Model file for the job. Use its own axes, mm. A direction names the side the tool comes from. Coordinates: 2 decimals unless noted, no trailing zeros. Write each loop counter-clockwise with the first axis right and the second up, starting at its lowest first coordinate (ties: lowest second). Pieces come first, ordered by that corner, then holes. Notation, with made-up numbers: (-16.75, 16.5) -> (-4.75, 16.5) arc R11 cw to (-4.75, 20.5) -> close; hole circle Ø4 at (59, 44). An arc over 180 degrees is marked (long way). Answer as a JSON object with one key per item and string values. Group by question number.
from build123d import *

# Parameters (mm, degrees)
SKETCH2_W                = 12.7
SKETCH2_H                = 12.7
BOSS_EXTRUDE4_DEPTH      = 3.6068
BOSS_EXTRUDE4_DEPTH_BACK = 2.7686
SKETCH3_W                = 1.000000006
SKETCH3_H                = 3.352800001
BOSS_EXTRUDE5_DEPTH      = 6.35
SKETCH4_R                = 0.79375
CUT_EXTRUDE1_DEPTH       = 10.854800007
SKETCH5_R                = 2.413000001
CUT_EXTRUDE2_DEPTH       = 2.54
SKETCH7_R                = 1.136382046
CUT_EXTRUDE4_DEPTH       = 7.3754


with BuildPart() as part:
    # Sketch2 → Boss-Extrude4 (new body, two sides)
    with BuildSketch(Plane(origin=(0, 0, 0), x_dir=(1, 0, 0), z_dir=(0, 1, 0))) as boss_extrude4_sk:
        with Locations((-0.031876663, -1.889989023)):
            Rectangle(SKETCH2_W, SKETCH2_H)
    extrude(amount=BOSS_EXTRUDE4_DEPTH)
    extrude(boss_extrude4_sk.sketch, amount=-BOSS_EXTRUDE4_DEPTH_BACK)

    # Sketch3 → Boss-Extrude5 (add)
    with BuildSketch(Plane.ZY.offset(6.381876663)):
        with Locations((-1.098810974, 0.417848354)):
            Rectangle(SKETCH3_W, SKETCH3_H)
        with Locations((4.894789026, 0.417848354)):
            Rectangle(SKETCH3_W, SKETCH3_H)
    extrude(amount=BOSS_EXTRUDE5_DEPTH)

    # Sketch4 → Cut-Extrude1 (cut, through all)
    with BuildSketch(Plane.XY.offset(5.394789029)):
        with Locations((-10.191876663, 0.417848354)):
            Circle(SKETCH4_R)
    extrude(amount=-CUT_EXTRUDE1_DEPTH, mode=Mode.SUBTRACT)

    # Sketch5 → Cut-Extrude2 (cut)
    with BuildSketch(Plane.XY.offset(8.239989023)):
        with Locations((-0.031876663, 0.417848354)):
            Circle(SKETCH5_R)
    extrude(amount=-CUT_EXTRUDE2_DEPTH, mode=Mode.SUBTRACT)

    # Sketch7 → Cut-Extrude4 (cut, through all)
    with BuildSketch(Plane(origin=(0, 3.6068, 0), x_dir=(1, 0, 0), z_dir=(0, 1, 0))):
        with Locations((-3.841876663, -1.89607107)):
            Circle(SKETCH7_R)
        with Locations((3.778123337, -1.89607107)):
            Circle(SKETCH7_R)
    extrude(amount=-CUT_EXTRUDE4_DEPTH, mode=Mode.SUBTRACT)


solid = part.part
(1) Cut at B-B on x = -9.75. List the corners of the cut face in (y, z).
(2) Cut at D-D on x = 4. List the corners of the cut face in (y, z).
(3) 3-axis set-ups, long thin cutter, end or side, ignore diameter. For faces 1 (the face through (-9, 0, 4.395)), 2 (the face through (0, 0, 5.7)), 3 (the face through (-9, 0, 5.395)), 4 (the face through (-10, -1.259, 5)), 5 (the face through (-9, 0, -1.599)): which of +Z, -Z, +X, -X, +Y, -Y reach the whole face in a straight line?
(4) Pull direction Y, two halves, no side cores. Call faces 6 (the face through (-10, 2.094, 5)), 7 (the face through (-2, 3, 8.24)), 8 (the face through (-10.985, 0.453, 4.902)): released by +Y, released by -Y, zero draft, split by the parting line, or undercut.
(5) Cut at C-C on z = 2.75. List the corners of the cut face in (x, y), plus the area to 3 significant figures.
(6) Cut at A-A on y = 0.75. List the corners of the cut face in (x, z), plus the area to 3 significant figures.
(7) Wall check: probe 1 along X at (y, z) = (-1.25, 2); probe 2 along Z at (x, y) = (-11.5, 2); probe 3 along X at (y, z) = (2.5, 1.5). Give the ranges that are in metal, low to high.
(8) Pin check, flat tips, straight feed: pin 1 (3.5 mm diameter, centred on x = -8.5, y = 0, fed in from +Z); pin 2 (1 mm diameter, centred on x = -10, y = 1, fed in from -Z); pin 3 (0.8 mm diameter, centred on x = -11, z = -1, fed in from +Y); pin 4 (3.5 mm diameter, centred on x = -3.84, z = 1.9, fed in from +Y). Stop position of each tip, or through.
Results found:
{
 "1": {"outline": "(-1.26, -1.6) -> (-0.24, -1.6) -> (-0.24, -0.6) -> (-1.26, -0.6) -> close; (-1.26, 4.39) -> (-0.24, 4.39) -> (-0.24, 5.39) -> (-1.26, 5.39) -> close; (1.08, -1.6) -> (2.09, -1.6) -> (2.09, -0.6) -> (1.08, -0.6) -> close; (1.08, 4.39) -> (2.09, 4.39) -> (2.09, 5.39) -> (1.08, 5.39) -> close"},
 "2": {"outline": "(-2.77, -4.46) -> (3.61, -4.46) -> (3.61, 0.78) -> (-2.77, 0.78) -> close; (-2.77, 3.01) -> (3.61, 3.01) -> (3.61, 8.24) -> (-2.77, 8.24) -> close"},
 "3": {"face 1": "-X, +Y, -Y", "face 2": "+Z", "face 3": "+Z, -X, +Y, -Y", "face 4": "+Z, -Z, -X, -Y", "face 5": "-Z, -X, +Y, -Y"},
 "4": {"face 6": "released by +Y", "face 7": "zero draft", "face 8": "undercut"},
 "5": {"outline": "(-6.38, -2.77) -> (-4.59, -2.77) -> (-4.59, 3.61) -> (-6.38, 3.61) -> close; (-3.09, -2.77) -> (3.03, -2.77) -> (3.03, 3.61) -> (-3.09, 3.61) -> close; (4.53, -2.77) -> (6.32, -2.77) -> (6.32, 3.61) -> (4.53, 3.61) -> close", "area": "61.8 mm²"},
 "6": {"outline": "(-12.73, -1.6) -> (-10.91, -1.6) -> (-10.91, -0.6) -> (-12.73, -0.6) -> close; (-12.73, 4.39) -> (-10.91, 4.39) -> (-10.91, 5.39) -> (-12.73, 5.39) -> close; (-9.47, -1.6) -> (-6.38, -1.6) -> (-6.38, -4.46) -> (6.32, -4.46) -> (6.32, 8.24) -> (2.36, 8.24) -> (2.36, 5.7) -> (-2.42, 5.7) -> (-2.42, 8.24) -> (-6.38, 8.24) -> (-6.38, 5.39) -> (-9.47, 5.39) -> (-9.47, 4.39) -> (-6.38, 4.39) -> (-6.38, -0.6) -> (-9.47, -0.6) -> close; hole circle Ø2.27 at (-3.84, 1.9); hole circle Ø2.27 at (3.78, 1.9)", "area": "151 mm²"},
 "7": {"probe 1": "x = -6.38 to -4.97, -2.71 to 2.65, 4.91 to 6.32", "probe 2": "z = -1.6 to -0.6, 4.39 to 5.39", "probe 3": "x = -6.38 to -4.91, -2.78 to 2.71, 4.84 to 6.32"},
 "8": {"pin 1": "stops at z = 5.39", "pin 2": "stops at z = -1.6", "pin 3": "stops at y = 2.09", "pin 4": "stops at y = 3.61"}
}
